For this review, take the finished solid that the model builds, in its own axes (mm). Round coordinates to 2 decimals unless told otherwise and drop trailing zeros. Write each loop counter-clockwise with the first axis right and the second up, starting at its lowest first coordinate (ties: lowest second). Pieces come first, ordered by that corner, then holes. Notation, with made-up numbers: (47, 57.5) - (74, 57.5) arc R8 cw to (74, 70.5) - close; hole circle Ø1 at (44, 88). An arc over 180 degrees is marked (long way). One line per item, written item: value. Start each with the question number.
Q1. For probe 1 along Y at (x, z) = (61, 6.15); probe 2 along Y at (x, z) = (10.5, 0); probe 3 along Y at (x, z) = (-46.5, 4.75), list the stretches that pass through material, from the lowest coordinate up.
Q2. Add section C-C on z = 1.75. Write out the cut boundary in (x, y).
Q3. Clearance check with a flat-ended pin moving along its axis: pin 1 Ø6 at (x, y) = (-45.5, 97.5) entering from -Z. State where the tip first meets the part, or that it passes through.
```python
from build123d import *

# Parameters (mm, degrees)
SKETCH_1_W          = 150
SKETCH_1_H          = 215
SKETCH_1_W_2        = 96
SKETCH_1_H_2        = 160
EXTRUDE_1_DEPTH     = 15
SKETCH_2_W          = 120
SKETCH_2_H          = 183
CUT_EXTRUDE_1_DEPTH = 5
CHAMFER_1_SIZE      = 5
SKETCH_5_W          = 130
SKETCH_5_H          = 190
CUT_EXTRUDE_2_DEPTH = 9
SKETCH_9_W          = 130
SKETCH_9_H          = 205
CUT_EXTRUDE_6_DEPTH = 4
SKETCH_10_R         = 2.5
CUT_EXTRUDE_7_DEPTH = 6
SKETCH_11_W         = 10
SKETCH_11_H         = 215
CUT_EXTRUDE_8_DEPTH = 5
EXTRUDE_2_DEPTH     = 3.5


with BuildPart() as part:
    # 草图1 → 凸台-拉伸1 (new body)
    with BuildSketch(Plane.XY):
        Rectangle(SKETCH_1_W, SKETCH_1_H)
        Rectangle(SKETCH_1_W_2, SKETCH_1_H_2, mode=Mode.SUBTRACT)
    extrude(amount=EXTRUDE_1_DEPTH)

    # 草图2 → 切除-拉伸1 (cut)
    with BuildSketch(Plane.XY.offset(15)):
        Rectangle(SKETCH_2_W, SKETCH_2_H)
    extrude(amount=-CUT_EXTRUDE_1_DEPTH, mode=Mode.SUBTRACT)

    # 倒角1
    chamfer_1_edges = [part.edges().sort_by_distance(p)[0] for p in [
        (0, -91.5, 15),
        (60, 0, 15),
        (-60, 0, 15),
        (0, 91.5, 15),
    ]]
    chamfer(chamfer_1_edges, length=CHAMFER_1_SIZE - 0.0001)  # a hair under: the kernel refuses the full size

    # 草图5 → 切除-拉伸2 (cut)
    with BuildSketch(Plane(origin=(0, 0, 0), x_dir=(-1, 0, 0), z_dir=(0, 0, -1))):
        Rectangle(SKETCH_5_W, SKETCH_5_H)
    extrude(amount=-CUT_EXTRUDE_2_DEPTH, mode=Mode.SUBTRACT)

    # 草图9 → 切除-拉伸6 (cut)
    with BuildSketch(Plane(origin=(0, 0, 0), x_dir=(-1, 0, 0), z_dir=(0, 0, -1))):
        Rectangle(SKETCH_9_W, SKETCH_9_H)
    extrude(amount=-CUT_EXTRUDE_6_DEPTH, mode=Mode.SUBTRACT)

    # 草图10 → 切除-拉伸7 (cut)
    with BuildSketch(Plane(origin=(0, 0, 4), x_dir=(-1, 0, 0), z_dir=(0, 0, -1))):
        with Locations((61, 98.5)):
            Circle(SKETCH_10_R)
        with Locations((-61, 98.5)):
            Circle(SKETCH_10_R)
        with Locations((-61, -98.5)):
            Circle(SKETCH_10_R)
        with Locations((61, -98.5)):
            Circle(SKETCH_10_R)
    extrude(amount=-CUT_EXTRUDE_7_DEPTH, mode=Mode.SUBTRACT)

    # 草图11 → 切除-拉伸8 (cut)
    with BuildSketch(Plane(origin=(0, 0, 0), x_dir=(-1, 0, 0), z_dir=(0, 0, -1))):
        Rectangle(SKETCH_11_W, SKETCH_11_H)
    extrude(amount=-CUT_EXTRUDE_8_DEPTH, mode=Mode.SUBTRACT)

    # 草图12 → 凸台-拉伸2 (add)
    with BuildSketch(Plane(origin=(0, 0, 0), x_dir=(-1, 0, 0), z_dir=(0, 0, -1))):
        Polygon((-5, 107.5), (-75, 107.5), (-75, -107.5), (-5, -107.5), (-5, -102.5), (-65, -102.5), (-65, 102.5), (-5, 102.5), align=None)
        Polygon((5, -102.5), (5, -107.5), (75, -107.5), (75, 107.5), (5, 107.5), (5, 102.5), (65, 102.5), (65, -102.5), align=None)
    extrude(amount=EXTRUDE_2_DEPTH)


solid = part.part
```
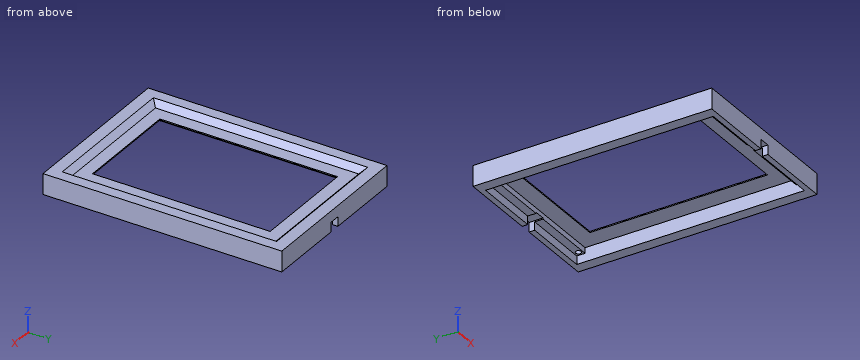
Result set:
1. probe 1: y = -107.5 to -101, -96 to -95, 95 to 96, 101 to 107.5
1. probe 2: y = -107.5 to -102.5, 102.5 to 107.5
1. probe 3: y = -107.5 to -95, 95 to 107.5
2. outline: (-75, -107.5) - (-5, -107.5) - (-5, -102.5) - (-65, -102.5) - (-65, 102.5) - (-5, 102.5) - (-5, 107.5) - (-75, 107.5) - close; (5, -107.5) - (75, -107.5) - (75, 107.5) - (5, 107.5) - (5, 102.5) - (65, 102.5) - (65, -102.5) - (5, -102.5) - close
3. pin 1: stops at z = 4
